Can you work these out from the model? Positions are in its coordinate system, mm. Round coordinates to 2 decimals unless told otherwise and drop trailing zeros. Order: outer loops, then holes, each group sorted by start corner. A loop starts at its lowest first (then second) coordinate and runs counter-clockwise, first axis right, second up. Notation, with made-up numbers: M 54.25,-5 L 73.25,-5 A29 ccw 73.25,23 Z; hole C 70.25,-22 d11. An arc over 180 degrees is marked long. Answer as a JSON object with one key per item and string values. Group by question number.
```python
from build123d import *

# Parameters (mm, degrees)
SKETCH_1_W          = 145
SKETCH_1_H          = 152
EXTRUDE_1_DEPTH     = 1
SKETCH_2_W          = 41
SKETCH_2_H          = 45
CUT_EXTRUDE_1_DEPTH = 1
SKETCH_3_R          = 1.6
CUT_EXTRUDE_2_DEPTH = 1
FILLET_1_R          = 3
SKETCH_7_R          = 1.55
CUT_EXTRUDE_6_DEPTH = 10


with BuildPart() as part:
    # 草图1 → 凸台-拉伸1 (new body)
    with BuildSketch(Plane.XY):
        Rectangle(SKETCH_1_W, SKETCH_1_H)
    extrude(amount=EXTRUDE_1_DEPTH)

    # 草图2 → 切除-拉伸1 (cut)
    with BuildSketch(Plane(origin=(0, 0, 0), x_dir=(-1, 0, 0), z_dir=(0, 0, -1))):
        with Locations((52, 14.5)):
            Rectangle(SKETCH_2_W, SKETCH_2_H)
        Polygon((-72.5, -31.894171459), (72.5, -70.746804361), (72.5, -76), (-72.5, -76), align=None)
    extrude(amount=-CUT_EXTRUDE_1_DEPTH, mode=Mode.SUBTRACT)

    # 草图3 → 切除-拉伸2 (cut)
    with BuildSketch(Plane.XY.offset(1)):
        with Locations((2.5, 71.5)):
            Circle(SKETCH_3_R)
        with Locations((22.5, 71.5)):
            Circle(SKETCH_3_R)
    extrude(amount=-CUT_EXTRUDE_2_DEPTH, mode=Mode.SUBTRACT)

    # 圆角1
    fillet_1_edges = [part.edges().sort_by_distance(p)[0] for p in [
        (72.5, -31.894171459, 0.5),
        (-72.5, -70.746804361, 0.5),
        (-72.5, -8, 0.5),
        (-31.5, -8, 0.5),
        (-31.5, 37, 0.5),
        (-72.5, 37, 0.5),
        (-72.5, 76, 0.5),
        (72.5, 76, 0.5),
    ]]
    fillet(fillet_1_edges, radius=FILLET_1_R)

    # 草图7 → 切除-拉伸6 (cut)
    with BuildSketch(Plane(origin=(0, 0, 0), x_dir=(-1, 0, 0), z_dir=(0, 0, -1))):
        with Locations((-69.5, 39.5)):
            Circle(SKETCH_7_R)
        with Locations((-69.5, 19.5)):
            Circle(SKETCH_7_R)
    extrude(amount=-CUT_EXTRUDE_6_DEPTH, mode=Mode.SUBTRACT)


solid = part.part
```
1) I need wall thicknesses on line 1 along X through (y, z) = (71.5, 0.5); line 2 along X through (y, z) = (2, 0.5); line 3 along Y through (x, z) = (69.5, 0.5). Which ranges of each line are inside material? Lowest first, please.
2) If we section it at A-A on z = 0.35: Write out the boundary of the cut face in (x, y).
3) For pin 1 (4 mm diameter, centred on x = 2.5, y = 71.5, fed in from -Z); pin 2 (0.5 mm diameter, centred on x = -56.5, z = 0.5, fed in from -Y), each with a flat end and sliding along its axis, tell me the tip position at first contact or that it passes through.
4) We'd pull the mould along X, two halves only. Please class faces 1 (the face through (-1, 4, 1)), 2 (the face through (1.75, -50.85, 0.49)), 3 (the face through (68.068, 38.906, 0.493)): +X half, -X half, draft (parallel to the pull), parting line (faces both ways), or undercut.
5) If we section it at C-C on y = -36: Write out the boundary of the cut face in (x, z), plus the area to 3 significant figures.
6) If we section it at B-B on x = -40: Write out the boundary of the cut face in (y, z), plus the area to 3 significant figures.
Findings:
{
 "1": {"line 1": "x = -72.5 to 0.9, 4.1 to 20.9, 24.1 to 72.5", "line 2": "x = -31.5 to 72.5", "line 3": "y = -32.7 to 17.95, 21.05 to 37.95, 41.05 to 76"},
 "2": {"outline": "M -72.5,-66.84 A3 ccw -68.72,-69.73 L 70.28,-32.49 A3 ccw 72.5,-29.59 L 72.5,73 A3 ccw 69.5,76 L -69.5,76 A3 ccw -72.5,73 L -72.5,40 A3 ccw -69.5,37 L -34.5,37 A3 cw -31.5,34 L -31.5,-5 A3 cw -34.5,-8 L -69.5,-8 A3 ccw -72.5,-11 Z; hole C 2.5,71.5 d3.2; hole C 22.5,71.5 d3.2; hole C 69.5,19.5 d3.1; hole C 69.5,39.5 d3.1"},
 "3": {"pin 1": "stops at z = 0", "pin 2": "stops at y = -66.53"},
 "4": {"face 1": "draft", "face 2": "+X half", "face 3": "undercut"},
 "5": {"outline": "M -72.5,0 L 57.18,0 L 57.18,1 L -72.5,1 Z", "area": "130 mm^2"},
 "6": {"outline": "M -62.04,0 L -8,0 L -8,1 L -62.04,1 Z; M 37,0 L 76,0 L 76,1 L 37,1 Z", "area": "93.0 mm^2"}
}
